Autodesk Inventor part; units mm, degrees
ref_plane "YZ Plane" through (0, 0, 0) normal (1, 0, 0) x (0, 1, 0)
ref_plane "XZ Plane" through (0, 0, 0) normal (0, 1, 0) x (-1, 0, 0)
ref_plane "XY Plane" through (0, 0, 0) normal (0, 0, 1) x (1, 0, 0)
sketch "Sketch1" plane through (0, 0, 0) normal (0, 0, 1) x (1, 0, 0)
  line L0 (6.5, 6.5) -> (-6.5, 6.5)
  line L1 (-6.5, 6.5) -> (-6.5, -6.5)
  line L2 (-6.5, -6.5) -> (6.5, -6.5)
  line L3 (6.5, -6.5) -> (6.5, 6.5)
  line L4 (6.5, 6.5) -> (-6.5, -6.5) construction
  line L5 (-6.5, 6.5) -> (6.5, -6.5) construction
  point P0 (0, 0)
  point P1 (0, 0)
  dimension "d35" = 13
  dimension "d36" = 13
extrude "Extrusion1" add sketch "Sketch1" along normal blind 3
sketch "Sketch2" plane through (0, 0, 0) normal (0, 0, -1) x (-1, 0, 0)
  line L0 (-6.5, 1) -> (6.5, 1)
  line L1 (6.5, 1) -> (6.5, -1)
  line L2 (6.5, -1) -> (-6.5, -1)
  line L3 (-6.5, -1) -> (-6.5, 1)
  line L4 (-6.5, 1) -> (6.5, -1) construction
  line L5 (6.5, 1) -> (-6.5, -1) construction
  circle A0 centre (0, 0) radius 4.9
  point P0 (4.7969, 1)
  point P1 (-4.7969, 1)
  point P2 (-4.7969, -1)
  point P3 (4.7969, -1)
  dimension "d3" = 2
  dimension "d4" = 13
  dimension "d57" = 9.8
extrude "Extrusion2" cut sketch "Sketch2" against normal blind 1.1 contours L0 A0 L2
sketch "Sketch22" plane through (6.5, -6.5, 0) normal (1, 0, 0) x (0, 0, -1)
  line L0 (0, 13) -> (-3, 13)
  line L1 (-3, 13) -> (-3, 0)
  line L2 (-3, 13) -> (-3, 0)
  line L3 (-3, 0) -> (-15, -17.1378)
  line L4 (-15, -17.1378) -> (-15, -9.1378)
  line L5 (-15, -9.1378) -> (-3, 13)
  line L6 (0, 0) -> (0, 13)
  point P0 (0, 6.5)
  point P1 (0, 6.5)
  dimension "d131" = 145
  dimension "d132" = 8
  dimension "d133" = 15
extrude "Extrusion20" add sketch "Sketch22" against normal blind 2
sketch "Sketch24" plane through (6.5, -6.5, 0) normal (1, 0, 0) x (0, 0, -1)
  circle A0 centre (-13, -10.5382) radius 1.25
  line L0 (0, 0) -> (0, 13)
  line L1 (-3, 13) -> (-15, -9.1378)
  line L2 (-15, -17.1378) -> (-3, 0)
  line L3 (-14.7588, -9.3067) -> (-11.2412, -11.7697) construction
  line L4 (-15, -17.1378) -> (-15, -9.1378)
  point P0 (0, 6.5)
  point P1 (0, 6.5)
  dimension "d141" = 2.5
  dimension "d142" = 13
  dimension "d149" = 90
extrude "Extrusion22" cut sketch "Sketch24" against normal blind 2
mirror "Mirror2" about plane through (0, 0, 0) normal (1, 0, 0) of "Extrusion20", "Extrusion22"
fillet "Fillet6" radius 2 10 edges at (-5.5, -23.6378, 15) (5.5, -23.6378, 15) (-6.5, -4.5689, 9) (6.5, -4.5689, 9) (-6.5, 6.5, 1.5) (-6.5, -15.0689, 9) (-6.5, -6.5, 1.5) (6.5, -15.0689, 9) (6.5, -6.5, 1.5) (6.5, 6.5, 1.5)
properties part number "PodstawkaKola"
Here's how the part is built. I have some questions about the finished solid (model axes, mm). A direction names the side the tool comes from. Give positions to 0.01 mm unless a question says otherwise; leave off trailing zeros. Write each loop counter-clockwise with the first axis right and the second up, starting at its lowest first coordinate (ties: lowest second). Pieces come first, ordered by that corner, then holes. Notation, with made-up numbers: (24.5, -35) -> (32.5, -35) arc R30 cw to (32.5, -12) -> close; hole circle Ø9 at (60, 83.25). An arc over 180 degrees is marked (long way). Use one line per item in the form item = value. Start each with the question number.
1. On a 3-axis mill with a long thin cutter (end or side, diameter ignored), from which of +Z, -Z, +X, -X, +Y, -Y can I reach the whole of each face in a straight line? I mean faces 1 (the face through (0, 0, 1.1)), 2 (the face through (4.5, -9, 8)), 3 (the face through (-5.9, -6.08, 9.17)). Say none if no direction works.
2. If I drill on L1, parallel to X at y = -5.75, z = 6.25; L2, parallel to Z at x = 0, y = 5; L3, parallel to X at y = -5.5, z = 9, over which ranges is the centre line in solid material (lowest first)?
3. Imagine slicing it at B-B on y = -16.75. State how many separate pieces and enclosed holes the cut face has, plus the area to 3 significant figures.
4. Imagine slicing it at A-A on x = -2.5. List the corners of the cut face in (y, z) for me.
5. Thinking about a two-plate mould opening in Y: for faces 4 (the face through (5, -17, 15)), 5 (the face through (5.93, -6.09, 9.14)), 6 (the face through (5.514, -15.984, 12.328)), which applies, +Y half, -Y half, draft (parallel to the pull), parting line (faces both ways), or undercut?
6. Will these pins go through, and if not, where does the flat tip stop? pin 1 Ø1 at (x, z) = (4.5, 10) entering from +Y; pin 2 Ø0.9 at (x, z) = (-1, 1.5) entering from -Y; pin 3 Ø4.5 at (x, y) = (-1, -0.5) entering from +Z.
Entries:
q1.face_1 = -Z
q1.face_2 = +Z, +Y, -Y
q1.face_3 = +Z, -X, +Y
q2.L1 = -6.5 to -4.5, 4.5 to 6.5
q2.L2 = 0 to 3
q2.L3 = -5.76 to -4.5, 4.5 to 5.76
q3.separate_pieces = 4
q3.enclosed_holes = 0
q3.area = 6.96 mm²
q4.outline = (-6.5, 0) -> (-1, 0) -> (-1, 1.1) -> (1, 1.1) -> (1, 0) -> (6.5, 0) -> (6.5, 3) -> (-6.5, 3) -> close
q5.face_4 = draft
q5.face_5 = +Y half
q5.face_6 = undercut
q6.pin_1 = -5.49
q6.pin_2 = -6.5
q6.pin_3 = 3
